The listing builds one solid part. Answer for the finished solid, in the listing's coordinates (mm). Coordinates: 2 decimals unless noted, no trailing zeros. Write each loop counter-clockwise with the first axis right and the second up, starting at its lowest first coordinate (ties: lowest second). Pieces come first, ordered by that corner, then holes.
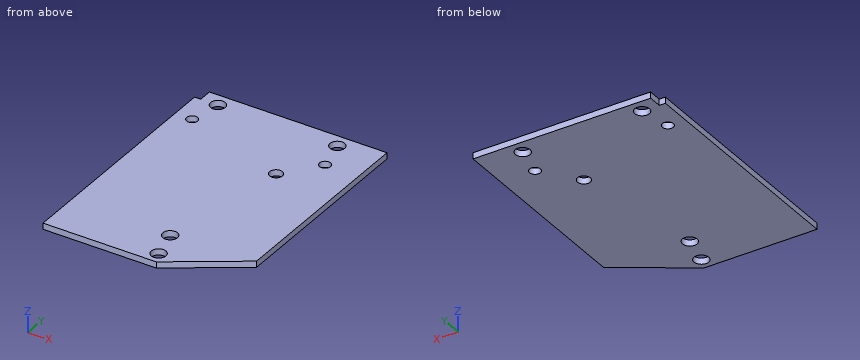
from build123d import *

# Parameters (mm, degrees)
F0_R     = 1.2
F0_R_2   = 0.9
F0_R_3   = 1.05
F1_DEPTH = 1


# Not quite as in the source:
# - a feature of the source that left no trace in its solid (it failed there, or was rolled back) is left out


with BuildPart() as f1:
    # F0 (on Top) → F1 (new body)
    with BuildSketch(Plane.XY):
        Polygon((27.5302478731, -17.7104764104), (27.5302478731, 15.4895235896), (-1.4697521269, 15.4895235896), (-1.4697521269, 13.2895235896), (-2.4697521269, 13.2895235896), (-2.4697521269, -22.3104764104), (-2.4697521269, -25.3104764104), (-1.4697521269, -25.3104764104), (16.0302478731, -25.3104764104), align=None)
        with Locations((15.1302478731, -23.3104764104)):
            Circle(F0_R, mode=Mode.SUBTRACT)
        with Locations((13.9302478731, -18.5104764104)):
            Circle(F0_R, mode=Mode.SUBTRACT)
        with Locations((0.3302478731, 8.2895235896)):
            Circle(F0_R_2, mode=Mode.SUBTRACT)
        with Locations((1.3302478731, 13.2895235896)):
            Circle(F0_R, mode=Mode.SUBTRACT)
        with Locations((17.6302478731, 2.6895235896)):
            Circle(F0_R_3, mode=Mode.SUBTRACT)
        with Locations((22.0302478731, 8.2895235896)):
            Circle(F0_R_2, mode=Mode.SUBTRACT)
        with Locations((20.8302478731, 13.2895235896)):
            Circle(F0_R, mode=Mode.SUBTRACT)
    extrude(amount=F1_DEPTH)


solid = f1.part
Q1. Find the intervals of material crossed by probe 1 along X at (y, z) = (9, 0.35); probe 2 along Y at (x, z) = (14.25, 0.3); probe 3 along Y at (x, z) = (16, 0.8), in increasing order.
Answers below:
probe 1: x = -2.47 to -0.22, 0.88 to 21.48, 22.58 to 27.53
probe 2: y = -25.31 to -24.13, -22.49 to -19.67, -17.35 to 15.49
probe 3: y = -25.31 to -24.14, -22.48 to 15.49
Q2. The part is cut by section A-A, the plane z = 0.25. Write down the section's boundary in (x, y).
Answers below:
outline: (-2.47, -25.31) - (16.03, -25.31) - (27.53, -17.71) - (27.53, 15.49) - (-1.47, 15.49) - (-1.47, 13.29) - (-2.47, 13.29) - close; hole circle Ø1.8 at (0.33, 8.29); hole circle Ø2.4 at (1.33, 13.29); hole circle Ø2.4 at (13.93, -18.51); hole circle Ø2.4 at (15.13, -23.31); hole circle Ø2.1 at (17.63, 2.69); hole circle Ø2.4 at (20.83, 13.29); hole circle Ø1.8 at (22.03, 8.29)
Q3. The part is cut by section B-B, the plane x = 1.75. Write down the section's boundary in (y, z), then the cut area to 3 significant figures.
Answers below:
outline: (-25.31, 0) - (12.17, 0) - (12.17, 1) - (-25.31, 1) - close; (14.41, 0) - (15.49, 0) - (15.49, 1) - (14.41, 1) - close
area: 38.6 mm2
